Input: part model. Units: mm. Frame: model coordinates. Round coordinates to 2 decimals unless told otherwise and drop trailing zeros. Loops run counter-clockwise (first coordinate to the right, second up) from the corner with the lowest first, then second, coordinate; pieces in that order, holes last. Notation, with made-up numbers: M 42,4 L 70,4 A19 cw 70,8 Z; hole C -26,87 d7. An arc over 180 degrees is marked long. Use one line per item in the form item = value. Start each with the question number.
Q1. First-contact query: P1, Ø1.5, axis at y = -1, z = 0, coming from the -X side; P2, Ø1, axis at x = 4.5, y = 0.5, coming from the +Z side. Flat tips, straight axial feed; report the tip coordinate or a pass-through.
Q2. Section query C-C, the plane z = 6.75. Output: boundary loops of the cut face in (x, y).
Q3. Section query D-D, the plane x = -1. Output: boundary loops of the cut face in (y, z).
Q4. Section query A-A, the plane z = -4.5. Output: boundary loops of the cut face in (x, y), and give its area (3 significant figures).
Q5. Section query B-B, the plane y = 0. Output: boundary loops of the cut face in (x, z).
Q6. Ray query, line 1 along X through (y, z) = (-0.2, 6.5); line 2 along Z through (x, y) = (2.75, 0.05); line 3 along Z through (x, y) = (-1, 0.5). Return the intervals inside material, ascending.
```python
from build123d import *

# Parameters (mm, degrees)
SKETCH2_R           = 1.5
RESISTOR_BODY_DEPTH = 8
LEAD1_PROFILE_R     = 0.35
SKETCH6_R           = 0.35
LEAD2_DEPTH         = 7


with BuildPart() as part:
    # Sketch2 → Resistor Body (new body)
    with BuildSketch(Plane.XY):
        Circle(SKETCH2_R)
    extrude(amount=RESISTOR_BODY_DEPTH)

    # Lead1: sweep along a path in Lead1 Path
    with BuildLine(Plane(origin=(0, 0, 0), x_dir=(1, 0, 0), z_dir=(0, 1, 0))) as lead1_path:
        Line((0, -8), (0, -10))
        ThreePointArc((0, -10), (0.585786438, -11.414213562), (2, -12))
        Line((2, -12), (3, -12))
        ThreePointArc((3, -12), (4.414213562, -11.414213562), (5, -10))
        Line((5, -10), (5, 7))
    # Lead1 Profile → Lead1 (sweep)
    with BuildSketch(Plane(origin=(0, 0, 8), x_dir=(-1, 0, 0), z_dir=(0, 0, 1))):
        Circle(LEAD1_PROFILE_R)
    sweep(path=lead1_path.line)

    # Sketch6 → Lead2 (add)
    with BuildSketch(Plane(origin=(0, 0, 0), x_dir=(1, 0, 0), z_dir=(0, 0, -1))):
        Circle(SKETCH6_R)
    extrude(amount=LEAD2_DEPTH)


solid = part.part
```
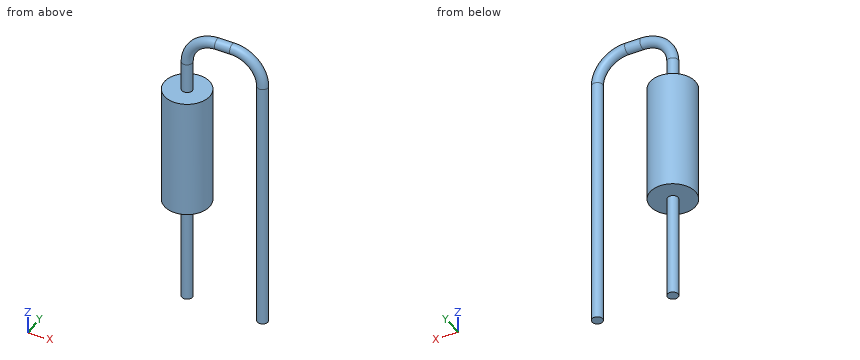
Results found:
q1.P1 = -1.48
q1.P2 = 12.01
q2.outline = C 0,0 d3; C 5,0 d0.7
q3.outline = M -1.12,0 L 1.12,0 L 1.12,8 L -1.12,8 Z
q4.outline = C 0,0 d0.7; C 5,0 d0.7
q4.area = 0.770 mm²
q5.outline = M -1.5,0 L -0.35,0 L -0.35,-7 L 0.35,-7 L 0.35,0 L 1.5,0 L 1.5,8 L 0.35,8 L 0.35,10 A1.65 cw 2,11.65 L 3,11.65 A1.65 cw 4.65,10 L 4.65,-7 L 5.35,-7 L 5.35,10 A2.35 ccw 3,12.35 L 2,12.35 A2.35 ccw -0.35,10 L -0.35,8 L -1.5,8 Z
q6.line_1 = -1.49 to 1.49, 4.71 to 5.29
q6.line_2 = 11.65 to 12.35
q6.line_3 = 0 to 8
